from build123d import *

# Parameters (mm, degrees)
BASE_FLANGE1_DEPTH = 1
CUT_EXTRUDE1_DEPTH = 10
CUT_EXTRUDE2_DEPTH = 10


# Sheet-metal steps are written as plain solids
with BuildPart() as part:
    # Sketch1 → Base-Flange1 (new body)
    with BuildSketch(Plane.XY):
        with BuildLine():
            Line((0, 0), (663.4, 0))
            Line((663.4, 0), (663.4, 992))
            ThreePointArc((663.4, 992), (658.801576465, 1003.101576465), (647.7, 1007.7))
            Line((647.7, 1007.7), (15.7, 1007.7))
            ThreePointArc((15.7, 1007.7), (4.598423535, 1003.101576465), (0, 992))
            Line((0, 992), (0, 0))
        make_face()
    extrude(amount=-BASE_FLANGE1_DEPTH)

    # Sketch9 → Cut-Extrude1 (cut)
    with BuildSketch(Plane.XY):
        with BuildLine():
            Line((562.2, 900.7), (301.2, 900.7))
            ThreePointArc((301.2, 900.7), (299.785786438, 900.114213562), (299.2, 898.7))
            Line((299.2, 898.7), (299.2, 814.7))
            ThreePointArc((299.2, 814.7), (299.785786438, 813.285786438), (301.2, 812.7))
            Line((301.2, 812.7), (562.2, 812.7))
            ThreePointArc((562.2, 812.7), (563.614213562, 813.285786438), (564.2, 814.7))
            Line((564.2, 814.7), (564.2, 898.7))
            ThreePointArc((564.2, 898.7), (563.614213562, 900.114213562), (562.2, 900.7))
        make_face()
        with BuildLine():
            Line((564.2, 718.7), (564.2, 634.7))
            ThreePointArc((564.2, 634.7), (563.614213562, 633.285786438), (562.2, 632.7))
            Line((562.2, 632.7), (301.2, 632.7))
            ThreePointArc((301.2, 632.7), (299.785786438, 633.285786438), (299.2, 634.7))
            Line((299.2, 634.7), (299.2, 718.7))
            ThreePointArc((299.2, 718.7), (299.785786438, 720.114213562), (301.2, 720.7))
            Line((301.2, 720.7), (562.2, 720.7))
            ThreePointArc((562.2, 720.7), (563.614213562, 720.114213562), (564.2, 718.7))
        make_face()
        with BuildLine():
            Line((564.2, 538.7), (564.2, 454.7))
            ThreePointArc((564.2, 454.7), (563.614213562, 453.285786438), (562.2, 452.7))
            Line((562.2, 452.7), (301.2, 452.7))
            ThreePointArc((301.2, 452.7), (299.785786438, 453.285786438), (299.2, 454.7))
            Line((299.2, 454.7), (299.2, 538.7))
            ThreePointArc((299.2, 538.7), (299.785786438, 540.114213562), (301.2, 540.7))
            Line((301.2, 540.7), (562.2, 540.7))
            ThreePointArc((562.2, 540.7), (563.614213562, 540.114213562), (564.2, 538.7))
        make_face()
        with BuildLine():
            Line((564.2, 358.7), (564.2, 274.7))
            ThreePointArc((564.2, 274.7), (563.614213562, 273.285786438), (562.2, 272.7))
            Line((562.2, 272.7), (301.2, 272.7))
            ThreePointArc((301.2, 272.7), (299.785786438, 273.285786438), (299.2, 274.7))
            Line((299.2, 274.7), (299.2, 358.7))
            ThreePointArc((299.2, 358.7), (299.785786438, 360.114213562), (301.2, 360.7))
            Line((301.2, 360.7), (562.2, 360.7))
            ThreePointArc((562.2, 360.7), (563.614213562, 360.114213562), (564.2, 358.7))
        make_face()
        with BuildLine():
            Line((564.2, 178.7), (564.2, 94.7))
            ThreePointArc((564.2, 94.7), (563.614213562, 93.285786438), (562.2, 92.7))
            Line((562.2, 92.7), (301.2, 92.7))
            ThreePointArc((301.2, 92.7), (299.785786438, 93.285786438), (299.2, 94.7))
            Line((299.2, 94.7), (299.2, 178.7))
            ThreePointArc((299.2, 178.7), (299.785786438, 180.114213562), (301.2, 180.7))
            Line((301.2, 180.7), (562.2, 180.7))
            ThreePointArc((562.2, 180.7), (563.614213562, 180.114213562), (564.2, 178.7))
        make_face()
    extrude(amount=-CUT_EXTRUDE1_DEPTH, mode=Mode.SUBTRACT)

    # Sketch10 → Cut-Extrude2 (cut)
    with BuildSketch(Plane.XY):
        with BuildLine():
            Line((66.2, 331.7), (198.2, 331.7))
            ThreePointArc((198.2, 331.7), (205.271067812, 334.628932188), (208.2, 341.7))
            Line((208.2, 341.7), (208.2, 889.2))
            ThreePointArc((208.2, 889.2), (205.271067812, 896.271067812), (198.2, 899.2))
            Line((198.2, 899.2), (66.2, 899.2))
            ThreePointArc((66.2, 899.2), (59.128932188, 896.271067812), (56.2, 889.2))
            Line((56.2, 889.2), (56.2, 341.7))
            ThreePointArc((56.2, 341.7), (59.128932188, 334.628932188), (66.2, 331.7))
        make_face()
    extrude(amount=-CUT_EXTRUDE2_DEPTH, mode=Mode.SUBTRACT)


solid = part.part
Design review of the part built by this model. Coordinates are the model's own, in mm. Give positions to 0.01 mm unless a question says otherwise; leave off trailing zeros. Order: outer loops, then holes, each group sorted by start corner. A loop starts at its lowest first (then second) coordinate and runs counter-clockwise, first axis right, second up.
1. Add section C-C, the plane x = 331.5. State the section outline as (y, z) points.
Solution:
outline: (0, -1) - (92.7, -1) - (92.7, 0) - (0, 0) - close; (180.7, -1) - (272.7, -1) - (272.7, 0) - (180.7, 0) - close; (360.7, -1) - (452.7, -1) - (452.7, 0) - (360.7, 0) - close; (540.7, -1) - (632.7, -1) - (632.7, 0) - (540.7, 0) - close; (720.7, -1) - (812.7, -1) - (812.7, 0) - (720.7, 0) - close; (900.7, -1) - (1007.7, -1) - (1007.7, 0) - (900.7, 0) - close
2. For pin 1 Ø0.5 at (x, z) = (477.5, -0.5) entering from -Y, flat-tipped, find the tip position at first contact; note if it passes through.
Solution:
pin 1: stops at y = 0
3. Add section A-A, the plane x = 160. State the section outline as (y, z) points.
Solution:
outline: (0, -1) - (331.7, -1) - (331.7, 0) - (0, 0) - close; (899.2, -1) - (1007.7, -1) - (1007.7, 0) - (899.2, 0) - close
4. Add section D-D, the plane z = -0.8. State how many separate pieces and enclosed holes the cut face has, then the cut area to 3 significant figures.
Solution:
separate pieces: 1
enclosed holes: 6
area: 466,000 mm2
5. To check wall thickness, follow L1, parallel to X at y = 872, z = -0.2; L2, parallel to Y at x = 360, z = -0.05; L3, parallel to X at y = 575.5, z = -0.5. State the ranges of each line that lie inside material, in increasing order.
Solution:
L1: x = 0 to 56.2, 208.2 to 299.2, 564.2 to 663.4
L2: y = 0 to 92.7, 180.7 to 272.7, 360.7 to 452.7, 540.7 to 632.7, 720.7 to 812.7, 900.7 to 1007.7
L3: x = 0 to 56.2, 208.2 to 663.4
6. Add section B-B, the plane y = 705.5. State the section outline as (x, z) points.
Solution:
outline: (0, -1) - (56.2, -1) - (56.2, 0) - (0, 0) - close; (208.2, -1) - (299.2, -1) - (299.2, 0) - (208.2, 0) - close; (564.2, -1) - (663.4, -1) - (663.4, 0) - (564.2, 0) - close
